```python
from build123d import *

# Parameters (mm, degrees)
PAD_DEPTH = 3


with BuildPart() as part:
    # Sketch → Pad (new body)
    with BuildSketch(Plane.XY):
        with BuildLine():
            ThreePointArc((-37.1, 50.8), (-37.807107, 50.507107), (-38.1, 49.8))
            Line((-38.1, -49.8), (-38.1, 49.8))
            ThreePointArc((-38.1, -49.8), (-37.807107, -50.507107), (-37.1, -50.8))
            Line((-37.1, -50.8), (-23.352, -50.8))
            ThreePointArc((-23.352, -50.8), (-22.644893, -50.507107), (-22.352, -49.8))
            Line((-22.352, -38.1), (-22.352, -49.8))
            ThreePointArc((-15.748, -38.1), (-19.05, -34.798), (-22.352, -38.1))
            Line((-15.748, -38.1), (-15.748, -49.8))
            ThreePointArc((-15.748, -49.8), (-15.455107, -50.507107), (-14.748, -50.8))
            Line((-14.748, -50.8), (14.748, -50.8))
            ThreePointArc((14.748, -50.8), (15.455107, -50.507107), (15.748, -49.8))
            Line((15.748, -38.1), (15.748, -49.8))
            ThreePointArc((22.352, -38.1), (19.05, -34.798), (15.748, -38.1))
            Line((22.352, -38.1), (22.352, -49.8))
            ThreePointArc((22.352, -49.8), (22.644893, -50.507107), (23.352, -50.8))
            Line((23.352, -50.8), (37.1, -50.8))
            ThreePointArc((37.1, -50.8), (37.807107, -50.507107), (38.1, -49.8))
            Line((38.1, 49.8), (38.1, -49.8))
            ThreePointArc((38.1, 49.8), (37.807107, 50.507107), (37.1, 50.8))
            Line((-37.1, 50.8), (37.1, 50.8))
        make_face()
    extrude(amount=PAD_DEPTH)


solid = part.part
```
Here's how the part is built. I have some questions about the finished solid (model axes, mm). A direction names the side the tool comes from. Coordinates: 2 decimals unless noted, no trailing zeros. Write each loop counter-clockwise with the first axis right and the second up, starting at its lowest first coordinate (ties: lowest second). Pieces come first, ordered by that corner, then holes. Notation, with made-up numbers: M 64.5,-8 L 83.5,-8 A24 cw 83.5,15 Z; hole C 44,-21.75 d9. An arc over 180 degrees is marked long. Answer as CSV lines item,"result". Start each with the question number.
Q1. Suppose I cut it at B-B, the plane z = 0.45. List the corners of the cut face in (x, y) for me.
Q2. Suppose I cut it at C-C, the plane x = 19.05. List the corners of the cut face in (y, z) for me.
Q3. For faces 1 (the flat face through (0, -50.8, 1)), 2 (the flat face through (22.352, -44, 1)), which set-ups out of +Z, -Z, +X, -X, +Y, -Y let a thin tool reach every point of the face, with its end or its side?
Q4. Suppose I cut it at A-A, the plane y = -37. List the corners of the cut face in (x, z) for me.
Q5. If we mould it in two halves opening along X, with no side actions, what happens to faces 3 (the flat face through (30, -50.8, 1)), 4 (the flat face through (-38.1, -1, 1)), 5 (the cylindrical face through (19.1, -34.8, 1.5))? For each: pulls with the +X half, pulls with the -X half, needs draft (parallel to the pull), parting line crosses it, or undercut.
Q6. I need wall thicknesses on probe 1 along X at (y, z) = (-41, 2.8); probe 2 along Y at (x, z) = (-19, 2.35); probe 3 along Y at (x, z) = (15, 0.3). Which ranges of each line are inside material? Lowest first, please. Write a range as [from, to].
Entries:
1,outline,"M -38.1,-49.8 A1 ccw -37.1,-50.8 L -23.35,-50.8 A1 ccw -22.35,-49.8 L -22.35,-38.1 A3.3 cw -15.75,-38.1 L -15.75,-49.8 A1 ccw -14.75,-50.8 L 14.75,-50.8 A1 ccw 15.75,-49.8 L 15.75,-38.1 A3.3 cw 22.35,-38.1 L 22.35,-49.8 A1 ccw 23.35,-50.8 L 37.1,-50.8 A1 ccw 38.1,-49.8 L 38.1,49.8 A1 ccw 37.1,50.8 L -37.1,50.8 A1 ccw -38.1,49.8 Z"
2,outline,"M -34.8,0 L 50.8,0 L 50.8,3 L -34.8,3 Z"
3,face 1,"+Z, -Z, +X, -X, -Y"
3,face 2,"+Z, -Z, -Y"
4,outline,"M -38.1,0 L -22.16,0 L -22.16,3 L -38.1,3 Z; M -15.94,0 L 15.94,0 L 15.94,3 L -15.94,3 Z; M 22.16,0 L 38.1,0 L 38.1,3 L 22.16,3 Z"
5,face 3,"needs draft"
5,face 4,"pulls with the -X half"
5,face 5,"undercut"
6,probe 1,"x = [-38.1, -22.35], [-15.75, 15.75], [22.35, 38.1]"
6,probe 2,"y = [-34.8, 50.8]"
6,probe 3,"y = [-50.77, 50.8]"
